The drawing under review shows one solid part. Ordinate dimensions are in mm from its lowest x, y, z. A direction names the side the tool comes from. Give positions to 0.01 mm unless a question says otherwise; leave off trailing zeros. Order: outer loops, then holes, each group sorted by start corner. A loop starts at its lowest first (then second) coordinate and runs counter-clockwise, first axis right, second up. Notation, with made-up numbers: (-35.5, -11.5) -> (-20.5, -11.5) arc R19 ccw to (-20.5, 5.5) -> close; hole circle Ø11 at (-19, 14). An arc over 180 degrees is marked (long way). Use CSV: the item, a comma, the result in double quotes. Start each with the question number.
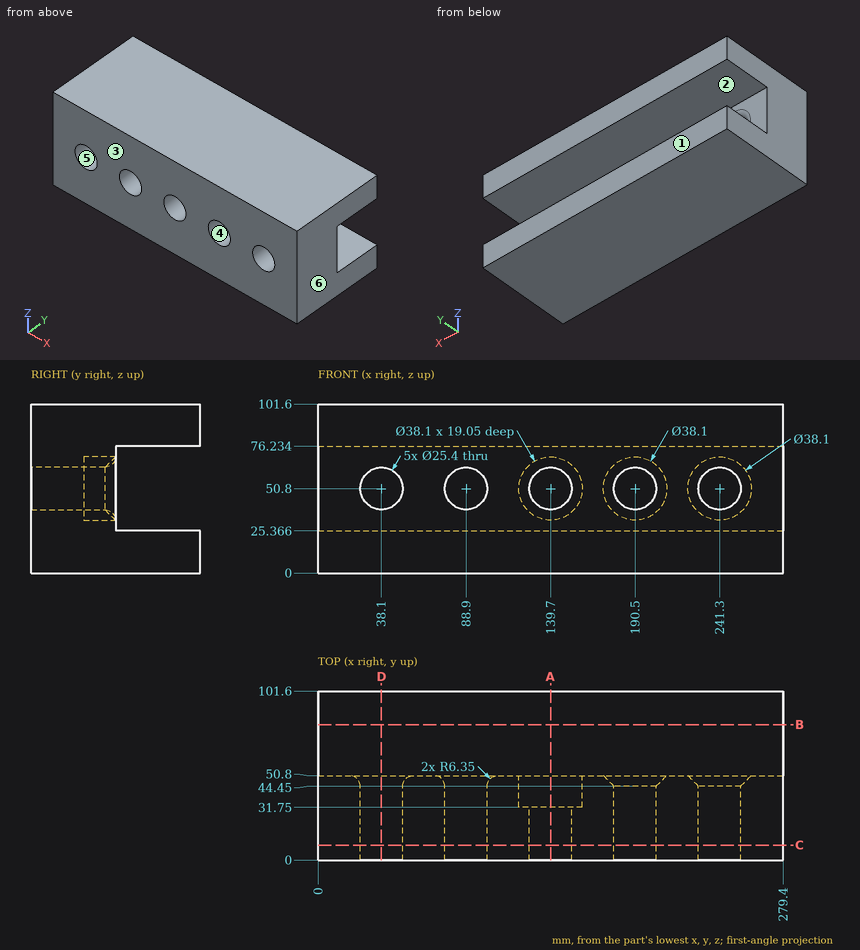
1. Clearance check with a flat-ended pin moving along its axis: P1, Ø15, axis at x = 88.9, z = 50.8, coming from the -Y side. State where the tip first meets the part, or that it passes through.
2. Draft analysis for pull direction X (two halves, no side actions). For the marked faces 3, 4, 5 and 6, state which applies: +X half, -X half, draft (parallel to the pull), parting line (faces both ways), or undercut.
3. Consider section C-C (y = 9). State the section outline as (x, z) points, plus the area to 3 significant figures.
4. Consider section D-D (x = 38.1). State the section outline as (y, z) points, plus the area to 3 significant figures.
5. To check wall thickness, follow L1, parallel to X at y = 40, z = 50; L2, parallel to Z at x = 241, y = 95; L3, parallel to Z at x = 139, y = 10. State the ranges of each line that lie inside material, in increasing order. Write a range as [from, to].
6. Consider section A-A (x = 139.7). State the section outline as (y, z) points.
7. Consider section B-B (y = 81.5). State the section outline as (x, z) points, plus the area to 3 significant figures.
8. For the marked faces 1 and 2, list the 3-axis set-ups (+Z, -Z, +X, -X, +Y, -Y) from which the entire face can be reached by the end or side of a thin tool; tool diameter is ignored.
Answer list:
1,P1,"through"
2,face 3,"draft"
2,face 4,"undercut"
2,face 5,"undercut"
2,face 6,"+X half"
3,outline,"(0, 0) -> (279.4, 0) -> (279.4, 101.6) -> (0, 101.6) -> close; hole circle Ø25.4 at (38.1, 50.8); hole circle Ø25.4 at (88.9, 50.8); hole circle Ø25.4 at (139.7, 50.8); hole circle Ø25.4 at (190.5, 50.8); hole circle Ø25.4 at (241.3, 50.8)"
3,area,"25,900 mm2"
4,outline,"(0, 0) -> (101.6, 0) -> (101.6, 25.37) -> (50.8, 25.37) -> (50.8, 31.75) arc R6.35 ccw to (44.45, 38.1) -> (0, 38.1) -> close; (0, 63.5) -> (44.45, 63.5) arc R6.35 ccw to (50.8, 69.85) -> (50.8, 76.23) -> (101.6, 76.23) -> (101.6, 101.6) -> (0, 101.6) -> close"
4,area,"6,430 mm2"
5,L1,"[0, 25.43], [50.77, 76.23], [101.57, 120.67], [158.73, 177.83], [203.17, 228.63], [253.97, 279.4]"
5,L2,"[0, 25.37], [76.23, 101.6]"
5,L3,"[0, 38.12], [63.48, 101.6]"
6,outline,"(0, 0) -> (101.6, 0) -> (101.6, 25.37) -> (50.8, 25.37) -> (50.8, 31.75) -> (31.75, 31.75) -> (31.75, 38.1) -> (0, 38.1) -> close; (0, 63.5) -> (31.75, 63.5) -> (31.75, 69.85) -> (50.8, 69.85) -> (50.8, 76.23) -> (101.6, 76.23) -> (101.6, 101.6) -> (0, 101.6) -> close"
7,outline,"(0, 0) -> (279.4, 0) -> (279.4, 25.37) -> (0, 25.37) -> close; (0, 76.23) -> (279.4, 76.23) -> (279.4, 101.6) -> (0, 101.6) -> close"
7,area,"14,200 mm2"
8,face 1,"+Z, -Z, +X, -X, +Y"
8,face 2,"+X, -X, +Y"
